The drawing under review shows one solid part. Ordinate dimensions are in mm from its lowest x, y, z. Coordinates: 2 decimals unless noted, no trailing zeros. Write each loop counter-clockwise with the first axis right and the second up, starting at its lowest first coordinate (ties: lowest second). Pieces come first, ordered by that corner, then holes.
1) To check wall thickness, follow line 1 along Y through (x, z) = (17.5, 1.85); line 2 along Y through (x, z) = (5.5, 1.95); line 3 along X through (y, z) = (5.75, 0.75). State the ranges of each line that lie inside material, in increasing order.
2) We need section D-D on y = 18.5. Write out the cut boundary in (x, z), then the cut area to 3 significant figures.
3) We need section C-C on x = 92.5. Write out the cut boundary in (y, z).
4) We need section A-A on z = 0.95. Give the number of separate pieces and of enclosed holes in the cut face, then the cut area to 3 significant figures.
5) Insertion check: P1, Ø1.5, axis at y = 15, z = 1, coming from the +X side; P2, Ø4.5, axis at x = 92.5, y = 10, coming from the -Z side. Each pin has a flat end and moves straight along its axis. Give the tip position at first contact, or say it passes through.
6) We need section B-B on x = 17.5. Write out the cut boundary in (y, z).
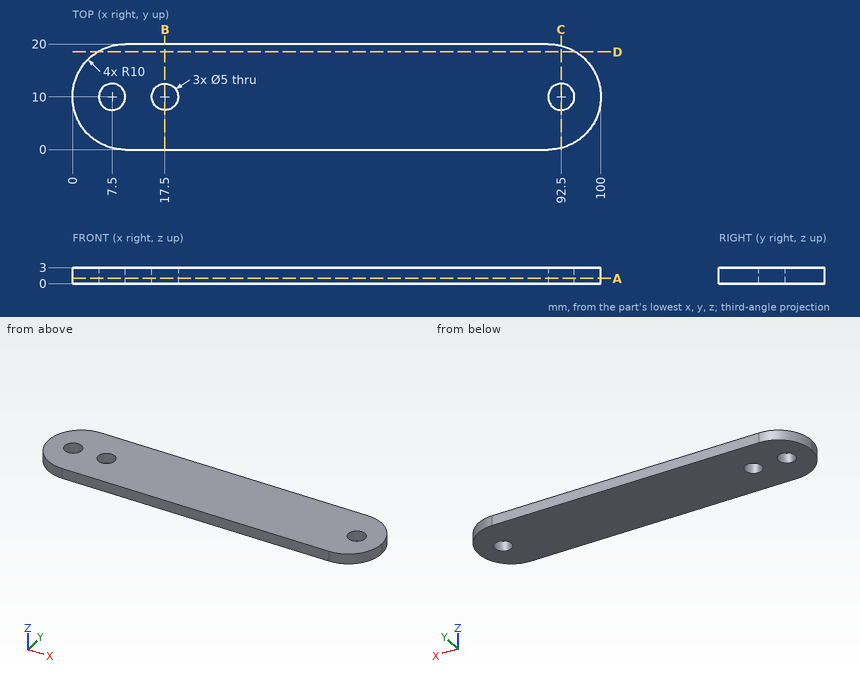
Result:
1. line 1: y = 0 to 7.5, 12.5 to 20
1. line 2: y = 1.07 to 8.5, 11.5 to 18.93
1. line 3: x = 0.95 to 99.05
2. outline: (4.73, 0) - (95.27, 0) - (95.27, 3) - (4.73, 3) - close
2. area: 272 mm2
3. outline: (0.32, 0) - (7.5, 0) - (7.5, 3) - (0.32, 3) - close; (12.5, 0) - (19.68, 0) - (19.68, 3) - (12.5, 3) - close
4. separate pieces: 1
4. enclosed holes: 3
4. area: 1,860 mm2
5. P1: stops at x = 99.05
5. P2: passes through
6. outline: (0, 0) - (7.5, 0) - (7.5, 3) - (0, 3) - close; (12.5, 0) - (20, 0) - (20, 3) - (12.5, 3) - close
